The listing builds one solid part. Answer for the finished solid, in the listing's coordinates (mm). A direction names the side the tool comes from. Give positions to 0.01 mm unless a question says otherwise; leave off trailing zeros. Loops run counter-clockwise (first coordinate to the right, second up) from the corner with the lowest first, then second, coordinate; pieces in that order, holes last.
Item 1: A tool of negligible diameter and unlimited length cuts with its end or side. For faces 1 (the face through (72, -15, 3)), 2 (the face through (72.719, -0.906, 2.8)), from which of +Z, -Z, +X, -X, +Y, -Y can it reach the whole face along a straight path? Write none if from no direction.
Item 2: Section D-D, the plane z = -104.5 is taken. Give the vertices of the cut face in (x, y), and give its area (3 significant figures).
Item 3: Each of these flat-tipped pins is pushed along its axis until it touches: pin 1 Ø6 at (x, z) = (-48, 55) entering from -Y; pin 2 Ø13 at (x, z) = (48, 55) entering from -Y; pin 3 Ø3 at (y, z) = (-1.5, -14) entering from -X. Where does it stop, or does it pass through?
Item 4: Section B-B, the plane y = -15.25 is taken. Give the vertices of the cut face in (x, z).
Item 5: Consider line 1 along Z through (x, y) = (48, 0); line 2 along X through (y, z) = (-13, 102); line 3 along Y through (x, z) = (41.5, -139.5). Determine where each line is inside the solid, lowest interval first.
Item 6: Section C-C, the plane x = -48 is taken. Give the vertices of the cut face in (y, z).
Item 7: The mould has two halves that part along Z. Classify faces 3 (the face through (-48.651, -0.021, 59.957)), 4 (the face through (17, -1, 200)), 5 (the face through (17, -1, -200)), 6 (the face through (-49.08, -0.02, 135.12)): pulls with the +Z half, pulls with the -Z half, needs draft (parallel to the pull), parting line crosses it, or undercut.
Item 8: Section A-A, the plane z = 140 is taken. Give the vertices of the cut face in (x, y).
Autodesk Inventor part; units mm, degrees
ref_plane "YZ Plane" through (0, 0, 0) normal (1, 0, 0) x (0, 1, 0)
ref_plane "XZ Plane" through (0, 0, 0) normal (0, 1, 0) x (-1, 0, 0)
ref_plane "XY Plane" through (0, 0, 0) normal (0, 0, 1) x (1, 0, 0)
sketch "Sketch4" plane through (0, 0, 0) normal (0, 1, 0) x (-1, 0, 0)
  line L0 (75, -200) -> (-75, -200)
  line L1 (-75, -200) -> (-75, 200)
  line L2 (-75, 200) -> (75, 200)
  line L3 (75, 200) -> (75, -200)
  line L4 (75, -200) -> (-75, 200) construction
  point P0 (0, 0)
  point P1 (0, 0)
  dimension "d24" = 150
  dimension "d25" = 400
extrude "Plate4" add sketch "Sketch4" along normal mid plane 3
sketch "Sketch7" plane through (0, -1.5, 0) normal (0, -1, 0) x (1, 0, 0)
  circle A0 centre (48, 55) radius 5
  line L0 (75, 200) -> (75, -200)
  line L1 (75, -200) -> (-75, -200)
  line L2 (0, -200) -> (0, 200) construction
  line L3 (75, 0) -> (-75, 0) construction
  circle A1 centre (-48, 55) radius 5
  circle A2 centre (48, 140) radius 5
  circle A3 centre (-48, 140) radius 5
  line L4 (75, 200) -> (-75, 200)
  point P0 (0, 0)
  point P1 (0, 0)
  dimension "d41" = 10
  dimension "d46" = 85
  dimension "d57" = 96
  dimension "d70" = 145
extrude "Extrusion2" cut sketch "Sketch7" against normal up to surface (3 mm away)
sketch "Sketch9" plane through (72, 1.5, -200) normal (1, 0, 0) x (0, -1, 0)
  line L0 (0, 400) -> (0, 0)
  line L1 (0, 0) -> (25, 0)
  line L2 (25, 0) -> (25, 400)
  line L3 (25, 400) -> (0, 400)
edge flange "Flange5" height 25 angle 90 thickness 3 bend radius 5 thickness toward (1, 0, 0) relief round relief width 3 relief depth 1.5 corner gap 5 corner form 0 edges at (75, 1.5, 0) (-75, 1.5, 0) wall of the first edge with corners at (72, 1.5, 200) (72, 1.5, -200) (72, -23.5, -200) (72, -23.5, 200)
bend "Bend5"
corner "Corner5"
sketch "Sketch12" plane through (0, 1.5, 0) normal (0, 1, 0) x (1, 0, 0)
  line L0 (-67, 200) -> (-67, -200)
  line L1 (67, -200) -> (-67, -200)
  line L2 (-56.875, -200) -> (-56.875, -81.7006) construction
  line L3 (-67, -150) -> (-26.2093, -150) construction
  circle A0 centre (-56.875, -150) radius 3
  point P0 (0, 0)
  dimension "d86" = 10.125
  dimension "d87" = 50
  dimension "d88" = 6
extrude "Extrusion5" [suppressed]
pattern_linear "Rectangular Pattern2" [suppressed]
equation "\"d25\" = Длина_базовой_пластины"
equation "\"d26\" = Thickness"
equation "\"d60\" = BendReliefWidth"
equation "\"d61\" = BendReliefDepth"
equation "\"d62\" = MinimumRemnant"
equation "\"d63\" = TransitionRadius"
equation "\"d66\" = BendRadius"
equation "\"d67\" = CornerReliefSize"
equation "\"d68\" = GapSize"
equation "\"d69\" = JacobiRadiusSize"
equation "\"BendReliefWidth\" = Thickness"
equation "\"BendReliefDepth\" = 0.5 * Thickness"
equation "\"CornerReliefSize\" = 4 * Thickness"
equation "\"MinimumRemnant\" = 2 * Thickness"
equation "\"TransitionRadius\" = BendRadius"
equation "\"JacobiRadiusSize\" = BendRadius"
equation "\"GapSize\" = Thickness"
properties part number "base plate 1" material "Stainless Steel"
Worked answers:
1. face 1: +Z, -Z, -Y
1. face 2: +Z, -Z, +X, +Y
2. outline: (-75, -23.5) - (-72, -23.5) - (-72, -6.5) arc R5 cw to (-67, -1.5) - (67, -1.5) arc R5 cw to (72, -6.5) - (72, -23.5) - (75, -23.5) - (75, -6.5) arc R8 ccw to (67, 1.5) - (-67, 1.5) arc R8 ccw to (-75, -6.5) - close
2. area: 565 mm2
3. pin 1: passes through
3. pin 2: stops at y = -1.5
3. pin 3: stops at x = -74.19
4. outline: (-75, -200) - (-72, -200) - (-72, 200) - (-75, 200) - close; (72, -200) - (75, -200) - (75, 200) - (72, 200) - close
5. line 1: z = -200 to 50, 60 to 135, 145 to 200
5. line 2: x = -75 to -72, 72 to 75
5. line 3: y = -1.5 to 1.5
6. outline: (-1.5, -200) - (1.5, -200) - (1.5, 50) - (-1.5, 50) - close; (-1.5, 60) - (1.5, 60) - (1.5, 135) - (-1.5, 135) - close; (-1.5, 145) - (1.5, 145) - (1.5, 200) - (-1.5, 200) - close
7. face 3: undercut
7. face 4: pulls with the +Z half
7. face 5: pulls with the -Z half
7. face 6: undercut
8. outline: (-75, -23.5) - (-72, -23.5) - (-72, -6.5) arc R5 cw to (-67, -1.5) - (-53, -1.5) - (-53, 1.5) - (-67, 1.5) arc R8 ccw to (-75, -6.5) - close; (-43, -1.5) - (43, -1.5) - (43, 1.5) - (-43, 1.5) - close; (53, -1.5) - (67, -1.5) arc R5 cw to (72, -6.5) - (72, -23.5) - (75, -23.5) - (75, -6.5) arc R8 ccw to (67, 1.5) - (53, 1.5) - close
